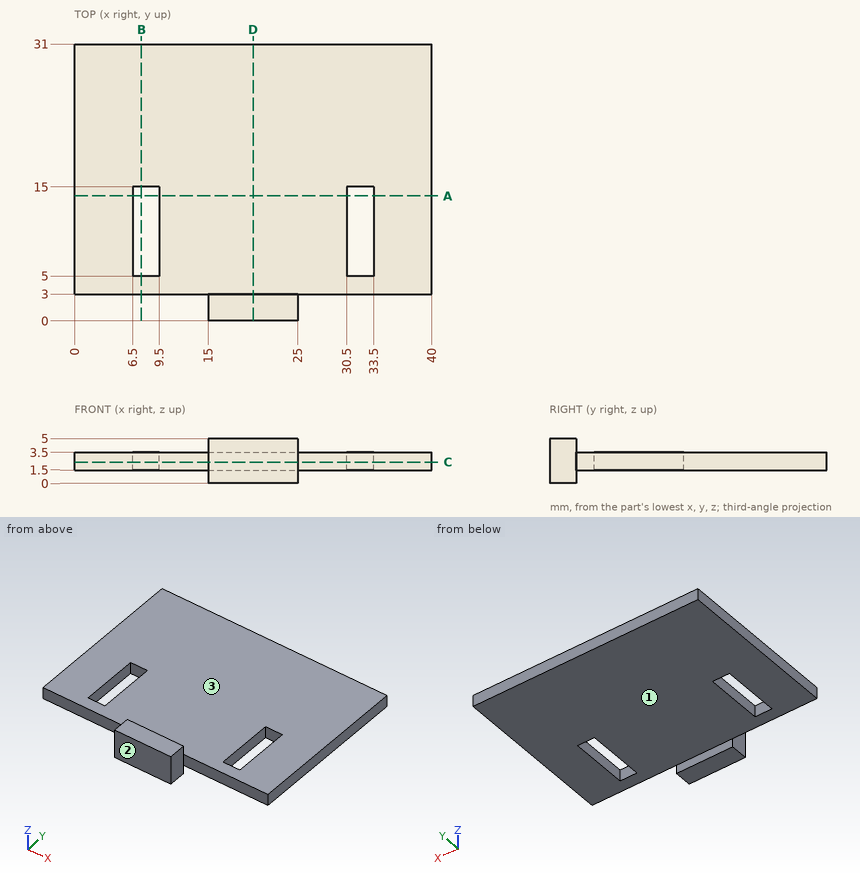
Check sheet for the drawn part. Datum: minimum x, y, z corner. Units: mm. A direction names the side the tool comes from. Round coordinates to 2 decimals unless told otherwise and drop trailing zeros. Order: outer loops, then holes, each group sorted by start corner. A loop starts at its lowest first (then second) coordinate and runs counter-clockwise, first axis right, second up.
(1) Cross-section at C-C, the plane z = 2.4. Enter the section's corners in (x, y), and give its area (3 significant figures).
(2) Cross-section at D-D, the plane x = 20. Enter the section's corners in (y, z).
(3) Cross-section at B-B, the plane x = 7.5. Enter the section's corners in (y, z).
(4) Scan lines: probe 1 along X at (y, z) = (10.5, 2.85); probe 2 along Z at (x, y) = (26.5, 13); probe 3 along Y at (x, z) = (23.5, 1.45). Record each from-to range of solid material in increasing order.
(5) Go/stop test with flat-tipped pins: P1, Ø5, axis at x = 31, y = 21, coming from the -Z side; P2, Ø1, axis at x = 28, y = 14, coming from the +Z side; P3, Ø2, axis at x = 7.5, z = 3, coming from the -Y side. Record where each tip stops, or that it passes through.
(6) Access from +Z, -Z, +X, -X, +Y, -Y to the whole of each face (thin tool, end or side, straight path). Record for the marked faces 1, 2 and 3.
(7) Cross-section at A-A, the plane y = 14. Enter the section's corners in (x, z).
Check sheet entries:
1. outline: (0, 3) - (15, 3) - (15, 0) - (25, 0) - (25, 3) - (40, 3) - (40, 31) - (0, 31) - close; hole (6.5, 5) - (9.5, 5) - (9.5, 15) - (6.5, 15) - close; hole (30.5, 5) - (33.5, 5) - (33.5, 15) - (30.5, 15) - close
1. area: 1,090 mm2
2. outline: (0, 0) - (3, 0) - (3, 1.5) - (31, 1.5) - (31, 3.5) - (3, 3.5) - (3, 5) - (0, 5) - close
3. outline: (3, 1.5) - (5, 1.5) - (5, 3.5) - (3, 3.5) - close; (15, 1.5) - (31, 1.5) - (31, 3.5) - (15, 3.5) - close
4. probe 1: x = 0 to 6.5, 9.5 to 30.5, 33.5 to 40
4. probe 2: z = 1.5 to 3.5
4. probe 3: y = 0 to 3
5. P1: stops at z = 1.5
5. P2: stops at z = 3.5
5. P3: stops at y = 3
6. face 1: -Z, +X, -X, +Y
6. face 2: +Z, -Z, +X, -X, -Y
6. face 3: +Z, +X, -X, +Y
7. outline: (0, 1.5) - (6.5, 1.5) - (6.5, 3.5) - (0, 3.5) - close; (9.5, 1.5) - (30.5, 1.5) - (30.5, 3.5) - (9.5, 3.5) - close; (33.5, 1.5) - (40, 1.5) - (40, 3.5) - (33.5, 3.5) - close
